Design review of the part built by this model. Coordinates are the model's own, in mm. A direction names the side the tool comes from. Coordinates: 2 decimals unless noted, no trailing zeros. Write each loop counter-clockwise with the first axis right and the second up, starting at its lowest first coordinate (ties: lowest second). Pieces come first, ordered by that corner, then holes. Notation, with made-up numbers: (38, 62.25) - (69, 62.25) arc R27 ccw to (69, 86.25) - close; hole circle Ø5 at (22, 33). An arc over 180 degrees is marked (long way). Answer as a JSON object with one key per item and string values.
Autodesk Inventor part; units mm, degrees
ref_plane "Work Plane1" through (0, 0, 0) normal (0, -1, 0) x (1, 0, 0)
ref_plane "YZ Plane" through (0, 0, 0) normal (1, 0, 0) x (0, 1, 0)
ref_plane "XZ Plane" through (0, 0, 0) normal (0, 1, 0) x (-1, 0, 0)
sketch "Sketch1" plane through (0, 0, 0) normal (0, 0, 1) x (1, 0, 0)
  line L0 (30.2, 0) -> (30.2, 5.65)
  line L1 (30.2, 5.65) -> (12, 5.65)
  arc A0 (12, 5.65) -> (10.15, 7.5) centre (10.15, 5.65) ccw
  line L2 (10.15, 7.5) -> (9, 7.5)
  line L3 (9, 7.5) -> (9, 8.5)
  line L4 (9, 8.5) -> (4.5, 10.5)
  line L5 (4.5, 10.5) -> (4.5, 20.5)
  line L6 (4.5, 20.5) -> (6.5, 20.5)
  line L7 (6.5, 20.5) -> (6.5, 23)
  line L8 (6.5, 23) -> (25.8, 23)
  line L9 (25.8, 23) -> (25.8, 26)
  line L10 (25.8, 26) -> (0, 26)
  line L11 (-6.04, 0) -> (36.24, 0)
  line L12 (0, 26) -> (0, 24.8)
  line L13 (0, 24.8) -> (0.5, 24.8)
  line L14 (2.5, 9) -> (6.5, 7.2222)
  line L15 (6.5, 7.2222) -> (6.5, 5)
  line L16 (6.5, 5) -> (5, 5)
  line L17 (5, 5) -> (5, 0)
  line L18 (0.5, 24.8) -> (0.5, 23)
  line L19 (0.5, 23) -> (2.5, 23)
  line L20 (2.5, 23) -> (2.5, 9)
  point P0 (0, 0)
  point P1 (21.1, 5.65)
  point P2 (0, 25.4)
  dimension "d2" = 11.3
  dimension "d3" = 52
  dimension "d4" = 15
  dimension "d5" = 3
  dimension "d6" = 7.5
  dimension "d7" = 25.8
  dimension "d8" = 21
  dimension "d9" = 1
  dimension "d10" = 18.2
  dimension "d11" = 3
  dimension "d12" = 1.2
  dimension "d13" = 0.5
  dimension "d14" = 10
  dimension "d15" = 1.5
  dimension "d16" = 5
  dimension "d17" = 30.2
  dimension "d18" = 18
  dimension "d19" = 2
  dimension "d20" = 41
  dimension "d23" = 2
revolve "Revolution1" add sketch "Sketch1" angle 360 about axis through (-10, 0, 0) along (1, 0, 0)
sketch "Sketch3" plane through (2.5, 0, 0) normal (-1, 0, 0) x (0, 0, 1)
  circle A0 centre (0, 0) radius 9
  circle A1 centre (0, 0) radius 23
  circle A2 centre (0, 0) radius 23
  line L0 (3, -22.8035) -> (4.5531, -13.1907)
  arc A3 (10.9475, -8.6532) -> (4.5531, -13.1907) centre (9.9827, -14.068) ccw
  line L1 (10.9475, -8.6532) -> (20.534, -10.3613)
  circle A4 centre (0, 0) radius 5.65 construction
  line L2 (9.9827, -14.068) -> (0, 0) construction
  line L3 (0, -36.4) -> (0, 36.4) construction
  line L4 (22.6145, -4.1935) -> (13.9521, 0.2542)
  arc A5 (11.6127, 7.7377) -> (13.9521, 0.2542) centre (16.4643, 5.1469) ccw
  line L5 (16.4643, 5.1469) -> (0, 0) construction
  line L6 (11.6127, 7.7377) -> (16.1995, 16.3272)
  line L7 (10.9765, 20.2118) -> (4.0697, 13.3478)
  arc A6 (-3.7705, 13.4354) -> (4.0697, 13.3478) centre (0.1927, 17.2489) ccw
  line L8 (0.1927, 17.2489) -> (0, 0) construction
  line L9 (-3.7705, 13.4354) -> (-10.5221, 20.452)
  line L10 (-15.8306, 16.6851) -> (-11.4369, 7.9952)
  arc A7 (-13.9429, 0.5658) -> (-11.4369, 7.9952) centre (-16.3451, 5.5135) ccw
  line L11 (-16.3451, 5.5135) -> (0, 0) construction
  line L12 (-13.9429, 0.5658) -> (-22.7025, -3.6871)
  line L13 (-20.7604, -9.8998) -> (-11.1381, -8.4065)
  arc A8 (-4.8468, -13.0857) -> (-11.1381, -8.4065) centre (-10.2946, -13.8414) ccw
  line L14 (-10.2946, -13.8414) -> (0, 0) construction
  line L15 (-4.8468, -13.0857) -> (-3.5088, -22.7308)
  circle A9 centre (0, 0) radius 11.75 construction
  circle A10 centre (0, 0) radius 23
  arc A11 (-15.8306, 16.6851) -> (-22.7025, -3.6871) centre (0, 0) ccw
  arc A12 (10.9765, 20.2118) -> (-10.5221, 20.452) centre (0, 0) ccw
  arc A13 (22.6145, -4.1935) -> (16.1995, 16.3272) centre (0, 0) ccw
  arc A14 (-20.7604, -9.8998) -> (-3.5088, -22.7308) centre (0, 0) ccw
  arc A15 (3, -22.8035) -> (20.534, -10.3613) centre (0, 0) ccw
  dimension "d24" = 3
  dimension "d25" = 21.5
  dimension "d28" = 360
  dimension "d30" = 23.5
  dimension "d31" = 5.5
extrude "Extrusion2" cut sketch "Sketch3" against normal blind 2 contours A1 L4 A5 L6 | L7 A6 L9 A1 | A1 L0 A3 L1 | L10 A7 L12 A1 | A1 L13 A8 L15
sketch "Sketch4" plane through (30.2, 0, 0) normal (1, 0, 0) x (0, 0, -1)
  line L0 (-1.825, 1.8519) -> (-1.825, -1.8519)
  line L1 (1.825, 1.8519) -> (1.825, -1.8519)
  arc A0 (-1.825, -1.8519) -> (1.825, -1.8519) centre (0, 0) ccw
  arc A1 (1.825, 1.8519) -> (-1.825, 1.8519) centre (0, 0) ccw
  dimension "d35" = 3.65
  dimension "d36" = 2.6
extrude "Extrusion3" cut sketch "Sketch4" against normal blind 13
ref_plane "Work Plane1" through (0, 0, 0) normal (0, -1, 0) x (1, 0, 0)
sketch "Sketch5" plane through (0, 0, 0) normal (0, -1, 0) x (1, 0, 0)
  line L0 (25.8, -26) -> (25.8, 26)
  line L1 (0, -26) -> (0, 26)
  line L2 (0, 26) -> (25.8, 26)
  line L3 (23.8, 26) -> (2, 26)
  line L4 (2, 26) -> (2, 24)
  line L5 (2, 24) -> (23.8, 24)
  line L6 (23.8, 24) -> (23.8, 26)
  line L7 (-6.04, 0) -> (36.24, 0)
  point P0 (0, 0)
  dimension "d40" = 2
  dimension "d41" = 2
  dimension "d42" = 2
revolve "Revolution2" cut sketch "Sketch5" angle 360 about axis through (-10, 0, 0) along (1, 0, 0) contours L6 L5 L4 L2
sketch "Sketch6" plane through (0, 0, 0) normal (0, 0, 1) x (1, 0, 0)
  line L0 (2, 24) -> (23.8, 24)
  line L1 (23.8, -26) -> (23.8, 26)
  line L2 (23.8, 26) -> (25.8, 26)
  line L3 (2, 26) -> (2, -26)
  line L4 (0, 26) -> (2, 26)
  arc A0 (2.6, 32.5) -> (0.1, 30) centre (2.6, 30) ccw
  line L5 (2.6, 32.5) -> (23.2, 32.5)
  arc A1 (25.7, 30) -> (23.2, 32.5) centre (23.2, 30) ccw
  line L6 (-6.6357, 0) -> (36.3393, 0)
  line L7 (0.1, 30) -> (0.1, 26)
  line L8 (25.7, 30) -> (25.7, 26)
  point P0 (0, 0)
  dimension "d44" = 65
  dimension "d45" = 2.5
  dimension "d46" = 0.1
  dimension "d47" = 0.1
revolve "Revolution3" add sketch "Sketch6" angle 360 about axis through (-10, 0, 0) along (1, 0, 0) contours L3 L4 L7 A0 L5 A1 L8 L2 L1 L0
scale "Scale1" factors (0.9, 0.9, 0.9) then translate (1.29, 0, 0) bodies 1
equation "\"d41\" = d40"
properties part number "velg"
(1) Take a section at B-B, the plane x = 15.5. Write out the cut boundary in (y, z) (3 decimals), and give its area (3 significant figures).
Solved:
{"outline": "circle Ø58.5 at (0, 0); circle Ø10.17 at (0, 0); hole circle Ø41.4 at (0, 0)", "area": "1,420 mm^2"}
(2) Tool access review of faces 4 (the face through (22.7, -2.34, 0.03)), 5 (the face through (4.427, -8.593, 6.165)), 6 (the face through (4.43, -16.26, 3.39)): name each direction out of +Z, -Z, +X, -X, +Y, -Y from which nothing blocks a thin tool from reaching the whole face with its end or side.
Solved:
{"face 4": "+X", "face 5": "+X, -X", "face 6": "-X"}
(3) The part is to be moulded in two halves that separate along Y. For faces 1 (the face through (4.427, -8.247, -14.415)), 2 (the face through (13.03, -6.341, -28.554)), 3 (the face through (1.29, 21, -9)), say which applies: pulls with the +Y half, pulls with the -Y half, needs draft (parallel to the pull), parting line crosses it, or undercut.
Solved:
{"face 1": "undercut", "face 2": "parting line crosses it", "face 3": "needs draft"}
(4) For pin 1 (3.5 mm diameter, centred on y = 19, z = 2, fed in from -X); pin 2 (10 mm diameter, centred on x = 20.5, y = 5.5, fed in from +Z); pin 3 (3 mm diameter, centred on y = -7, z = -15.5, fed in from -X), all flat-tipped, find the tip position at first contact; note any pin that passes through.
Solved:
{"pin 1": "stops at x = 1.74", "pin 2": "stops at z = 29.25", "pin 3": "stops at x = 3.54"}
(5) Take a section at C-C, the plane y = -16.5. Give the number of separate pieces and of enclosed holes in the cut face, and give its area (3 significant figures).
Solved:
{"separate pieces": "3", "enclosed holes": "0", "area": "559 mm^2"}
(6) Take a section at A-A, the plane x = 23.5. Write out the cut boundary in (y, z) (1 decimal), and give its area (3 significant figures).
Solved:
{"outline": "circle Ø57.6 at (0, 0); circle Ø10.2 at (0, 0); hole circle Ø41.4 at (0, 0); hole (-1.7, -1.6) - (1.7, -1.6) arc R2.3 ccw to (1.7, 1.6) - (-1.7, 1.6) arc R2.3 ccw to start", "area": "1,330 mm^2"}
(7) To check wall thickness, follow line 1 (Z direction, x = 5.9, y = 0); line 2 (Z direction, x = 6.5, y = 0); line 3 (Y direction, x = 10, z = -1). State the ranges of each line that lie inside material, in increasing order. Write a range as from..to.
Solved:
{"line 1": "z = -29.25..-18.45, -9.2..-7.05, -4.5..4.5, 7.05..9.2, 18.45..29.25", "line 2": "z = -29.25..-18.45, -8.93..-6.78, -4.5..4.5, 6.78..8.93, 18.45..29.25", "line 3": "y = -29.23..-20.68, -6.68..6.68, 20.68..29.23"}
